Input: dimensioned drawing with shaded views. Units: mm. Origin: part minimum x, y, z. Give positions to 0.01 mm unless a question says otherwise; leave off trailing zeros. Loops run counter-clockwise (first coordinate to the right, second up) from the corner with the lowest first, then second, coordinate; pieces in that order, holes last. Notation, with made-up numbers: M 53,14.5 L 91,14.5 A24 ccw 91,53.5 Z; hole C -6,28.5 d5. An arc over 180 degrees is marked long. Answer in a Markdown table with one row per item.
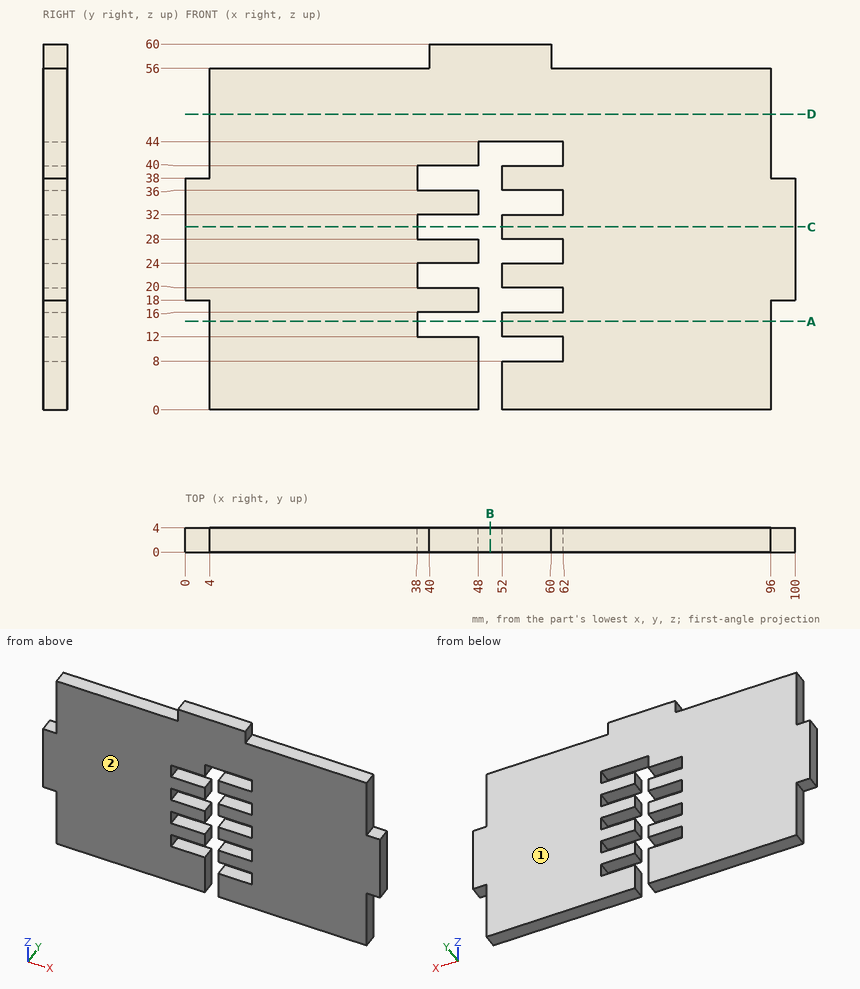
Q1. Contact query for flat-ended pins moving along their axis: pin 1 Ø1.5 at (y, z) = (2.5, 43.5) entering from -X; pin 2 Ø1.2 at (y, z) = (2.5, 57.5) entering from +X; pin 3 Ø1.2 at (x, y) = (1.5, 2.5) entering from +Z. Output: stop coordinate, or through.
Values follow:
| item | result |
|---|---|
| pin 1 | x = 4 |
| pin 2 | x = 60 |
| pin 3 | z = 38 |
Q2. Section query C-C (z = 30). Output: boundary loops of the cut face in (x, y), plus the area to 3 significant figures.
Values follow:
| item | result |
|---|---|
| outline | M 0,0 L 38,0 L 38,4 L 0,4 Z; M 52,0 L 100,0 L 100,4 L 52,4 Z |
| area | 344 mm^2 |
Q3. Ray query, probe 1 along Z at (x, y) = (43.5, 1); probe 2 along Z at (x, y) = (61, 0.75); probe 3 along Z at (x, y) = (55, 2). Return the intervals inside material, ascending. Write a range as from..to.
Values follow:
| item | result |
|---|---|
| probe 1 | 0..12, 16..20, 24..28, 32..36, 40..60 |
| probe 2 | 0..8, 12..16, 20..24, 28..32, 36..40, 44..56 |
| probe 3 | 0..8, 12..16, 20..24, 28..32, 36..40, 44..60 |
Q4. Section query D-D (z = 48.5). Output: boundary loops of the cut face in (x, y), plus the area to 3 significant figures.
Values follow:
| item | result |
|---|---|
| outline | M 4,0 L 96,0 L 96,4 L 4,4 Z |
| area | 368 mm^2 |
Q5. Section query A-A (z = 14.5). Output: boundary loops of the cut face in (x, y), plus the area to 3 significant figures.
Values follow:
| item | result |
|---|---|
| outline | M 4,0 L 38,0 L 38,4 L 4,4 Z; M 52,0 L 96,0 L 96,4 L 52,4 Z |
| area | 312 mm^2 |
Q6. Mould query, pull axis Y, two halves, no side actions, for the marked faces 1 and 2. Classes: +Y half, -Y half, draft (parallel to the pull), parting line (faces both ways), or undercut.
Values follow:
| item | result |
|---|---|
| face 1 | +Y half |
| face 2 | -Y half |
Q7. Section query B-B (x = 50). Output: boundary loops of the cut face in (y, z).
Values follow:
| item | result |
|---|---|
| outline | M 0,44 L 4,44 L 4,60 L 0,60 Z |
